Autodesk Inventor part; units mm, degrees
ref_plane "YZ Plane" through (0, 0, 0) normal (1, 0, 0) x (0, 1, 0)
ref_plane "XZ Plane" through (0, 0, 0) normal (0, 1, 0) x (-1, 0, 0)
ref_plane "XY Plane" through (0, 0, 0) normal (0, 0, 1) x (1, 0, 0)
sketch "Sketch1" plane through (0, 0, 0) normal (0, 0, 1) x (1, 0, 0)
  line L0 (40, 32.5) -> (-40, 32.5)
  line L1 (-40, 32.5) -> (-40, -32.5)
  line L2 (-40, -32.5) -> (40, -32.5)
  line L3 (40, -32.5) -> (40, 32.5)
  line L4 (40, 32.5) -> (-40, -32.5) construction
  line L5 (-40, 32.5) -> (40, -32.5) construction
  line L6 (-33, 29) -> (33, 29) construction
  line L7 (33, 29) -> (33, -29) construction
  line L8 (33, -29) -> (-33, -29) construction
  line L9 (-33, -29) -> (-33, 29) construction
  line L10 (-33, 29) -> (33, -29) construction
  line L11 (33, 29) -> (-33, -29) construction
  line L12 (40, 0) -> (-40, 0) construction
  line L13 (0, 32.5) -> (0, -32.5) construction
  circle A0 centre (33, 29) radius 2.4
  circle A1 centre (-33, 29) radius 2.4
  circle A2 centre (33, -29) radius 2.4
  circle A3 centre (-33, -29) radius 2.4
  line L14 (33, 32.25) -> (33, 25.75) construction
  arc A4 (35.2895, 28.2801) -> (35.2895, 29.7199) centre (35.5, 29) ccw
  arc A5 (30.7105, 29.7199) -> (30.7105, 28.2801) centre (30.5, 29) ccw
  arc A6 (-35.2895, 29.7199) -> (-35.2895, 28.2801) centre (-35.5, 29) ccw
  arc A7 (-30.7105, 28.2801) -> (-30.7105, 29.7199) centre (-30.5, 29) ccw
  arc A8 (35.2895, -29.7199) -> (35.2895, -28.2801) centre (35.5, -29) ccw
  arc A9 (30.7105, -28.2801) -> (30.7105, -29.7199) centre (30.5, -29) ccw
  arc A10 (-35.2895, -28.2801) -> (-35.2895, -29.7199) centre (-35.5, -29) ccw
  arc A11 (-30.7105, -29.7199) -> (-30.7105, -28.2801) centre (-30.5, -29) ccw
  line L15 (39, 25.5) -> (-39, 25.5)
  line L16 (-39, 25.5) -> (-39, -25.5)
  line L17 (-39, -25.5) -> (39, -25.5)
  line L18 (39, -25.5) -> (39, 25.5)
  line L19 (39, 25.5) -> (-39, -25.5) construction
  line L20 (-39, 25.5) -> (39, -25.5) construction
  point P0 (0, 0)
  point P1 (36.25, 29)
  point P2 (29.75, 29)
  point P3 (36.25, -29)
  point P4 (30.7105, 28.2801)
  point P5 (30.7105, 29.7199)
  point P6 (-30.7105, 29.7199)
  point P7 (-30.7105, 28.2801)
  point P8 (-35.2895, 28.2801)
  point P9 (-35.2895, 29.7199)
  point P10 (-30.7105, -28.2801)
  point P11 (-30.7105, -29.7199)
  point P12 (-35.2895, -29.7199)
  point P13 (-35.2895, -28.2801)
  point P14 (35.2895, -28.2801)
  point P15 (35.2895, -29.7199)
  point P16 (30.7105, -29.7199)
  point P17 (30.7105, -28.2801)
  dimension "d0" = 80
  dimension "d1" = 65
  dimension "d19" = 4.8
  dimension "d30" = 6.5
  dimension "d33" = 58
  dimension "d34" = 66
  dimension "d35" = 6.5
  dimension "d36" = 1.5
  dimension "d37" = 7
  dimension "d38" = 1
  dimension "d39" = 51
  dimension "d40" = 78
  dimension "d41" = 14
extrude "Extrusion1" add sketch "Sketch1" along normal blind 1.6 contours L3 L2 L1 L0 | L18 L17 L16 L15
extrude "Extrusion2" add sketch "Sketch1" along normal blind 16.6 contours L18 L17 L16 L15
fillet "Fillet1" radius 2 4 edges at (39, -25.5, 9.1) (39, 25.5, 9.1) (-39, -25.5, 9.1) (-39, 25.5, 9.1)
properties part number "SUSTAINA-ACTUATOR-POWER-BOARD" material "Acetal Resin, Black"
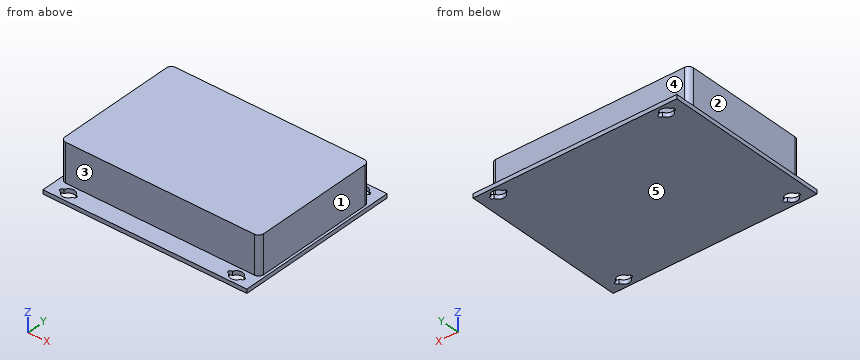
Can you work these out from the model? Positions are in its coordinate system, mm. Face numbers are marked on the shaded views. A direction names the side the tool comes from. Coordinates: 2 decimals unless noted, no trailing zeros. Order: outer loops, then holes, each group sorted by start corner. A loop starts at its lowest first (then second) coordinate and runs counter-clockwise, first axis right, second up. Notation, with made-up numbers: (42, 48.5) -> (100, 48.5) arc R32 cw to (100, 86.5) -> close; hole circle Ø3 at (82, 72.25). An arc over 180 degrees is marked (long way). Write each question's results on one line, items separated by ' | '.
Item 1: I want a section at B-B, the plane x = -23. Write out the boundary of the cut face in (y, z).
Results are:
outline: (-32.5, 0) -> (32.5, 0) -> (32.5, 1.6) -> (25.5, 1.6) -> (25.5, 16.6) -> (-25.5, 16.6) -> (-25.5, 1.6) -> (-32.5, 1.6) -> close
Item 2: If I drill on line 1 along Y through (x, z) = (-35.5, 0.7); line 2 along Y through (x, z) = (0, 8); line 3 along X through (y, z) = (-3, 5.75), over which ranges is the centre line in solid material (lowest first)?
Results are:
line 1: -32.5 to -29.75, -28.25 to 28.25, 29.75 to 32.5 | line 2: -25.5 to 25.5 | line 3: -39 to 39
Item 3: Which directions (+Z, -Z, +X, -X, +Y, -Y) give clear straight access to the entire face, cutting with the end or side of a thin tool? Please do the marked faces 1, 2, 3, 4 and 5.
Results are:
face 1: +Z, +X, +Y, -Y | face 2: +Z, -X, +Y, -Y | face 3: +Z, +X, -X, -Y | face 4: +Z, +X, -X, +Y | face 5: -Z, +X, -X, +Y, -Y
Item 4: I want a section at A-A, the plane z = 5. Write out the boundary of the cut face in (x, y).
Results are:
outline: (-39, -23.5) arc R2 ccw to (-37, -25.5) -> (37, -25.5) arc R2 ccw to (39, -23.5) -> (39, 23.5) arc R2 ccw to (37, 25.5) -> (-37, 25.5) arc R2 ccw to (-39, 23.5) -> close
Item 5: I want a section at C-C, the plane x = -33.5. Write out the boundary of the cut face in (y, z).
Results are:
outline: (-32.5, 0) -> (-31.35, 0) -> (-31.35, 1.6) -> (-32.5, 1.6) -> close; (-26.65, 0) -> (26.65, 0) -> (26.65, 1.6) -> (25.5, 1.6) -> (25.5, 16.6) -> (-25.5, 16.6) -> (-25.5, 1.6) -> (-26.65, 1.6) -> close; (31.35, 0) -> (32.5, 0) -> (32.5, 1.6) -> (31.35, 1.6) -> close
Item 6: I'm going to push flat-ended pins straight in: pin 1 Ø2 at (x, z) = (24.5, 7) entering from -Y; pin 2 Ø2.5 at (x, y) = (35.5, -29) entering from +Z; pin 3 Ø7.5 at (y, z) = (-3.5, 6) entering from -X. Where does each tip first touch, or does it pass through?
Results are:
pin 1: y = -25.5 | pin 2: z = 1.6 | pin 3: x = -39
